Source: three-view drawing plus pictorial views. Frame: mm from the lowest corner of the part. A direction names the side the tool comes from. Coordinates: 2 decimals unless noted, no trailing zeros. Order: outer loops, then holes, each group sorted by start corner. A loop starts at its lowest first (then second) coordinate and runs counter-clockwise, first axis right, second up. Notation, with made-up numbers: (-7, 9.5) - (12, 9.5) arc R13 ccw to (12, 17.5) - close; hole circle Ø3 at (4, 61). An arc over 180 degrees is marked (long way). One line per question, with ' | ' between items.
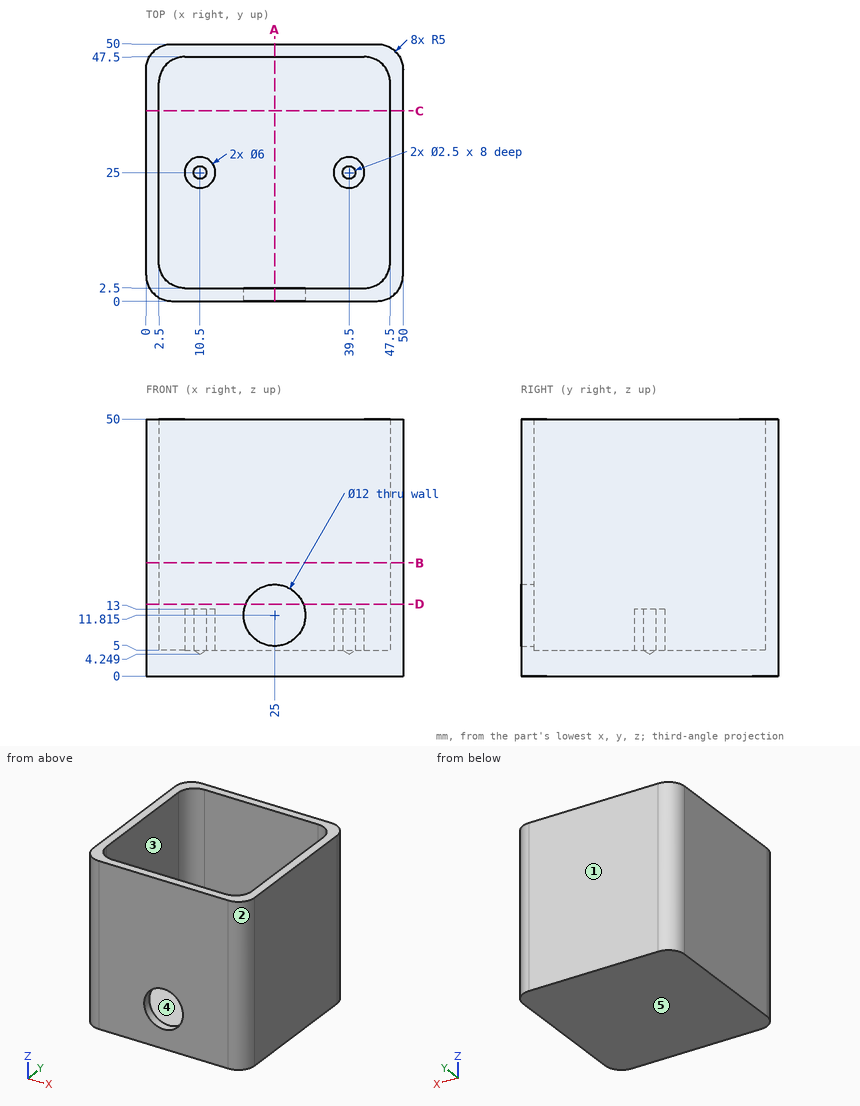
Item 1: Section D-D on z = 14. Return the cut outline in (x, y), and give its area (3 significant figures).
Data:
outline: (0, 5) arc R5 ccw to (5, 0) - (19.41, 0) - (19.41, 2.5) - (7.5, 2.5) arc R5 cw to (2.5, 7.5) - (2.5, 42.5) arc R5 cw to (7.5, 47.5) - (42.5, 47.5) arc R5 cw to (47.5, 42.5) - (47.5, 7.5) arc R5 cw to (42.5, 2.5) - (30.59, 2.5) - (30.59, 0) - (45, 0) arc R5 ccw to (50, 5) - (50, 45) arc R5 ccw to (45, 50) - (5, 50) arc R5 ccw to (0, 45) - close | area: 447 mm^2
Item 2: Access query for the marked faces 4 and 5. Directions: +Z, -Z, +X, -X, +Y, -Y. A direction counts if a zero-diameter tool reaches every point of the face in a straight line with its end or side. Return the directions, or none.
Data:
face 4: +Z | face 5: -Z, +X, -X, +Y, -Y
Item 3: Section A-A on x = 25. Return the cut outline in (y, z) (1 decimal), and give its area (3 significant figures).
Data:
outline: (0, 0) - (50, 0) - (50, 50) - (47.5, 50) - (47.5, 5) - (2.5, 5) - (2.5, 5.8) - (0, 5.8) - close; (0, 17.8) - (2.5, 17.8) - (2.5, 50) - (0, 50) - close | area: 445 mm^2
Item 4: Section B-B on z = 22. Return the cut outline in (x, y), and give its area (3 significant figures).
Data:
outline: (0, 5) arc R5 ccw to (5, 0) - (45, 0) arc R5 ccw to (50, 5) - (50, 45) arc R5 ccw to (45, 50) - (5, 50) arc R5 ccw to (0, 45) - close; hole (2.5, 7.5) arc R5 ccw to (7.5, 2.5) - (42.5, 2.5) arc R5 ccw to (47.5, 7.5) - (47.5, 42.5) arc R5 ccw to (42.5, 47.5) - (7.5, 47.5) arc R5 ccw to (2.5, 42.5) - close | area: 475 mm^2
Item 5: Draft query along X for the marked faces 1, 2 and 3. Return one class per face: released by +X, released by -X, zero draft, split by the parting line, or undercut.
Data:
face 1: zero draft | face 2: released by +X | face 3: undercut
Item 6: Ray query, line 1 (Y direction, x = 10.5, z = 8.25); line 2 (X direction, y = 28, z = 19). Return the intervals inside material, ascending.
Data:
line 1: 0 to 2.5, 22 to 23.75, 26.25 to 28, 47.5 to 50 | line 2: 0 to 2.5, 47.5 to 50
Item 7: Contact query for flat-ended pins moving along their axis: P1, Ø6.5, axis at x = 40.5, y = 24, coming from the +Z side; P2, Ø3, axis at x = 17.5, y = 44, coming from the +Z side; P3, Ø2, axis at x = 10.5, y = 25, coming from the +Z side. Output: stop coordinate, or through.
Data:
P1: z = 13 | P2: z = 5 | P3: z = 4.85
Item 8: Section C-C on y = 37. Return the cut outline in (x, z), and give its area (3 significant figures).
Data:
outline: (0, 0) - (50, 0) - (50, 50) - (47.5, 50) - (47.5, 5) - (2.5, 5) - (2.5, 50) - (0, 50) - close | area: 475 mm^2
